Part model, mm, in its own coordinate system. Face numbers are marked on the shaded views. Give positions to 0.01 mm unless a question says otherwise; leave off trailing zeros. Order: outer loops, then holes, each group sorted by start corner. A loop starts at its lowest first (then second) coordinate and runs counter-clockwise, first axis right, second up. Notation, with made-up numbers: (-5.5, -15.75) -> (42.5, -15.75) arc R22 ccw to (42.5, -3.75) -> close; hole circle Ø6 at (80.25, 46.25). An arc over 180 degrees is marked (long way). Write item = value, one per line. Start each with the question number.
(1) Saw through at C-C, the plane y = 43.5. List the corners of the cut face in (x, z).
(2) Saw through at D-D, the plane y = -32.5. List the corners of the cut face in (x, z), then the cut area to 3 significant figures.
(3) Probe line 1 along X through (y, z) = (81, -225); line 2 along X through (y, z) = (-3, -225); line 3 along X through (y, z) = (77.5, -292.5). List the from-to ranges inside material, lowest first. Write a range as from..to.
(4) Two-plate mould, pull along Z, no slides. Class the marked faces 1, 2 and 3: pulls with the +Z half, pulls with the -Z half, needs draft (parallel to the pull), parting line crosses it, or undercut.
(5) Saw through at B-B, the plane x = 0. List the corners of the cut face in (y, z), then the cut area to 3 significant figures.
(6) Flat gauge pins, fed straight in: pin 1 (8 mm diameter, centred on x = 37, y = -26.5, fed in from +Z); pin 2 (6 mm diameter, centred on y = 74, z = -104, fed in from +X); pin 3 (4 mm diameter, centred on x = -53.5, y = 46.5, fed in from +Z); pin 4 (5 mm diameter, centred on x = 57.5, z = -2, fed in from -Y). Where does each tip first touch, or does it go through?
(7) Saw through at A-A, the plane z = -225. List the corners of the cut face in (x, y).
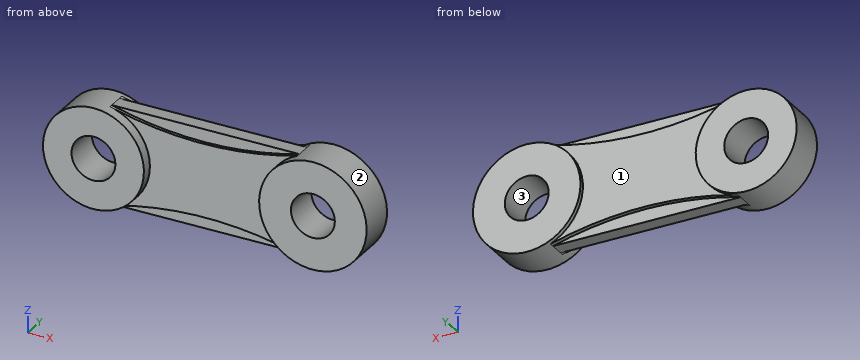
from build123d import *

# Parameters (mm, degrees)
CROQUIS3_W                   = 1000
CROQUIS3_H                   = 450
SALIENTE_EXTRUIR4_DEPTH      = 100
SALIENTE_EXTRUIR5_DEPTH      = 20
SALIENTE_EXTRUIR5_DEPTH_BACK = 150
CROQUIS6_R                   = 245
CROQUIS6_R_2                 = 230
CORTAR_EXTRUIR5_DEPTH        = 20
CORTAR_EXTRUIR4_DEPTH        = 1342.575566265
CORTAR_EXTRUIR4_DEPTH_BACK   = 1342.575566265
CROQUIS8_R                   = 100
CORTAR_EXTRUIR6_START        = -15
CORTAR_EXTRUIR6_DEPTH        = 15


with BuildPart() as part:
    # Croquis3 → Saliente-Extruir4 (new body)
    with BuildSketch(Plane(origin=(0, 0, 0), x_dir=(1, 0, 0), z_dir=(0, 1, 0))):
        with Locations((500, 225)):
            Rectangle(CROQUIS3_W, CROQUIS3_H)
    extrude(amount=SALIENTE_EXTRUIR4_DEPTH)

    # Croquis6 → Saliente-Extruir5 (add, two sides: drawn at the far end of the back side and taken through both)
    with BuildSketch(Plane(origin=(0, 100, 0), x_dir=(1, 0, 0), z_dir=(0, 1, 0)).offset(-SALIENTE_EXTRUIR5_DEPTH_BACK)):
        with Locations(Location((1000, 225, 0), (0, 0, 270))):
            Circle(CROQUIS6_R)
        with Locations(Location((0, 225, 0), (0, 0, 270))):
            Circle(CROQUIS6_R_2)
    extrude(amount=SALIENTE_EXTRUIR5_DEPTH + SALIENTE_EXTRUIR5_DEPTH_BACK)

    # Croquis7 → Cortar-Extruir5 (cut)
    with BuildSketch(Plane(origin=(0, 100, 0), x_dir=(1, 0, 0), z_dir=(0, 1, 0))):
        with BuildLine():
            Line((47.696960071, 0), (903.046402852, 0))
            ThreePointArc((903.046402852, 0), (475.371681461, 58.217157741), (47.696960071, 0))
        make_face()
        with BuildLine():
            Line((47.696960071, 450), (903.046402852, 450))
            ThreePointArc((903.046402852, 450), (475.371681461, 391.782842259), (47.696960071, 450))
        make_face()
    extrude(amount=-CORTAR_EXTRUIR5_DEPTH, mode=Mode.SUBTRACT)

    # Croquis8 → Cortar-Extruir4 (cut, two sides: drawn at the far end of the back side and taken through both)
    with BuildSketch(Plane(origin=(0, 120, 0), x_dir=(1, 0, 0), z_dir=(0, 1, 0)).offset(-CORTAR_EXTRUIR4_DEPTH_BACK)):
        with Locations(Location((0, 225, 0), (0, 0, 270))):
            Circle(CROQUIS8_R)
        with Locations(Location((1000, 225, 0), (0, 0, 270))):
            Circle(CROQUIS8_R)
    extrude(amount=CORTAR_EXTRUIR4_DEPTH + CORTAR_EXTRUIR4_DEPTH_BACK, mode=Mode.SUBTRACT)

    # Croquis9 → Cortar-Extruir6 (cut)
    with BuildSketch(Plane.XZ.offset(CORTAR_EXTRUIR6_START)):
        with BuildLine():
            Line((47.696960071, 0), (903.046402852, 0))
            ThreePointArc((903.046402852, 0), (475.371681461, -58.217157741), (47.696960071, 0))
        make_face()
        with BuildLine():
            Line((47.696960071, -450), (903.046402852, -450))
            ThreePointArc((903.046402852, -450), (475.371681461, -391.782842259), (47.696960071, -450))
        make_face()
    extrude(amount=CORTAR_EXTRUIR6_DEPTH, mode=Mode.SUBTRACT)


solid = part.part
Results list:
q1.outline = (47.7, -450) -> (903.05, -450) arc R245 ccw (long way) to (903.05, 0) -> (47.7, 0) arc R230 ccw (long way) to start; hole circle Ø200 at (0, -225); hole circle Ø200 at (1000, -225)
q2.outline = circle Ø460 at (0, -225); circle Ø490 at (1000, -225); hole circle Ø200 at (0, -225); hole circle Ø200 at (1000, -225)
q2.area = 292,000 mm^2
q3.line_1 = -230..-100, 100..900, 1100..1245
q3.line_2 = -230..-100, 100..230, 755..900, 1100..1245
q3.line_3 = -219.87..-73.78, 73.78..926.22, 1073.78..1235.52
q4.face_1 = needs draft
q4.face_2 = parting line crosses it
q4.face_3 = undercut
q5.outline = (-50, -455) -> (120, -455) -> (120, -325) -> (-50, -325) -> close; (-50, -125) -> (120, -125) -> (120, 5) -> (-50, 5) -> close
q5.area = 44,200 mm^2
q6.pin_1 = 2.62
q6.pin_2 = 1214.71
q6.pin_3 = -0.84
q6.pin_4 = -50
q7.outline = (-230, -50) -> (-100, -50) -> (-100, 120) -> (-230, 120) -> close; (100, -50) -> (230, -50) -> (230, 0) -> (755, 0) -> (755, -50) -> (900, -50) -> (900, 120) -> (755, 120) -> (755, 100) -> (230, 100) -> (230, 120) -> (100, 120) -> close; (1100, -50) -> (1245, -50) -> (1245, 120) -> (1100, 120) -> close
